from build123d import *

# Parameters (mm, degrees)
SKETCH1_W           = 266
SKETCH1_H           = 7
SKETCH1_R           = 1.8
SKETCH1_W_2         = 15
SKETCH1_H_2         = 166.79
BOSS_EXTRUDE1_DEPTH = 5
SKETCH2_W           = 266
SKETCH2_H           = 9.605
BOSS_EXTRUDE2_DEPTH = 5
SKETCH3_W           = 17.215
SKETCH3_H           = 12.5
SKETCH3_W_2         = 0.785
BOSS_EXTRUDE3_DEPTH = 2
FILLET1_R           = 0.5
FILLET2_R           = 50
FILLET3_R           = 2
FILLET4_R           = 100


with BuildPart() as part:
    # Sketch1 → Boss-Extrude1 (new body)
    # profile 1 of 4: a face of its own
    with BuildSketch(Plane.YZ):
        with Locations((0, 86.895)):
            Rectangle(SKETCH1_W, SKETCH1_H)
        with Locations(Location((113.375, 86.895, 0), (0, 0, 270))):
            Circle(SKETCH1_R, mode=Mode.SUBTRACT)
        with Locations(Location((-113.375, 86.895, 0), (0, 0, 270))):
            Circle(SKETCH1_R, mode=Mode.SUBTRACT)
    # profile 2 of 4: a face of its own
    with BuildSketch(Plane.YZ):
        with Locations((125.5, 0)):
            Rectangle(SKETCH1_W_2, SKETCH1_H_2)
    # profile 3 of 4: a face of its own
    with BuildSketch(Plane.YZ):
        with Locations((-125.5, 0)):
            Rectangle(SKETCH1_W_2, SKETCH1_H_2)
    # profile 4 of 4: a face of its own
    with BuildSketch(Plane.YZ):
        with Locations((0, -86.895)):
            Rectangle(SKETCH1_W, SKETCH1_H)
        with Locations(Location((-113.375, -86.895, 0), (0, 0, 270))):
            Circle(SKETCH1_R, mode=Mode.SUBTRACT)
        with Locations(Location((113.375, -86.895, 0), (0, 0, 270))):
            Circle(SKETCH1_R, mode=Mode.SUBTRACT)
    extrude(amount=BOSS_EXTRUDE1_DEPTH)

    # Sketch2 → Boss-Extrude2 (add)
    with BuildSketch(Plane.YZ.offset(5)):
        with Locations((0, 95.1975)):
            Rectangle(SKETCH2_W, SKETCH2_H)
        with Locations((0, -95.1975)):
            Rectangle(SKETCH2_W, SKETCH2_H)
    extrude(amount=-BOSS_EXTRUDE2_DEPTH)

    # Sketch3 → Boss-Extrude3 (add)
    # profile 1 of 2: a face of its own
    with BuildSketch(Plane(origin=(0, 0, -100), x_dir=(1, 0, 0), z_dir=(0, 0, -1))):
        with Locations((-3.6075, 139.25)):
            Rectangle(SKETCH3_W, SKETCH3_H)
        with BuildLine():
            ThreePointArc((-4.215, 136.45), (-7.015, 139.25), (-4.215, 142.05))
            Line((-4.215, 142.05), (-2.215, 142.05))
            ThreePointArc((-2.215, 142.05), (0.585, 139.25), (-2.215, 136.45))
            Line((-2.215, 136.45), (-4.215, 136.45))
        make_face(mode=Mode.SUBTRACT)
    # profile 2 of 2: a face of its own
    with BuildSketch(Plane(origin=(0, 0, -100), x_dir=(1, 0, 0), z_dir=(0, 0, -1))):
        with Locations((5.3925, 139.25)):
            Rectangle(SKETCH3_W_2, SKETCH3_H)
    extrude(amount=-BOSS_EXTRUDE3_DEPTH)

    # Fillet1
    fillet1_edges = [part.edges().sort_by_distance(p)[0] for p in [
        (2.5, -133, -98),
    ]]
    fillet(fillet1_edges, radius=FILLET1_R)

    # Fillet2
    # the kernel refuses this fillet: 50 mm, written as the material it adds along each edge
    with BuildSketch(Plane(origin=(0, -133, -100), x_dir=(0, 1, 0), z_dir=(0, 0, 1))) as fillet2_piece_1:
        with BuildLine():
            CenterArc((32.745897071, 50), FILLET2_R, 229.086571868, 40.913428132)
            Line((0, 12.215), (0, 0))
            Line((0, 0), (32.745897071, 0))
        make_face()
    extrude(amount=2)

    # Fillet3
    fillet3_edges = [part.edges().sort_by_distance(p)[0] for p in [
        (-12.215, -145.5, -99),
        (5.785, -145.5, -99),
    ]]
    fillet(fillet3_edges, radius=FILLET3_R)

    # Mirror1: part across plane


with BuildPart() as part_1:
    add(part.part)
    add(part.part.mirror(Plane.XY))

    # Mirror2: part across plane


with BuildPart() as part_2:
    add(part_1.part)
    add(part_1.part.mirror(Plane.ZX))

    # Fillet4
    # the kernel refuses this fillet: 100 mm, written as the material it adds along each edge
    with BuildSketch(Plane(origin=(5, 133, 98), x_dir=(1, 0, 0), z_dir=(0, 0, 1)), Plane(origin=(5, 133, -100), x_dir=(1, 0, 0), z_dir=(0, 0, 1)), Plane(origin=(5, -133, -98), x_dir=(1, 0, 0), z_dir=(0, 0, -1)), Plane(origin=(5, -133, 100), x_dir=(1, 0, 0), z_dir=(0, 0, -1))) as fillet4_piece_1:
        with BuildLine():
            CenterArc((100, -12.505349855), FILLET4_R, 172.816154735, 7.183845265)
            Line((0, -12.505349855), (0, 0))
            Line((0, 0), (0.785, 0))
        make_face()
    extrude(amount=2)


solid = part_2.part
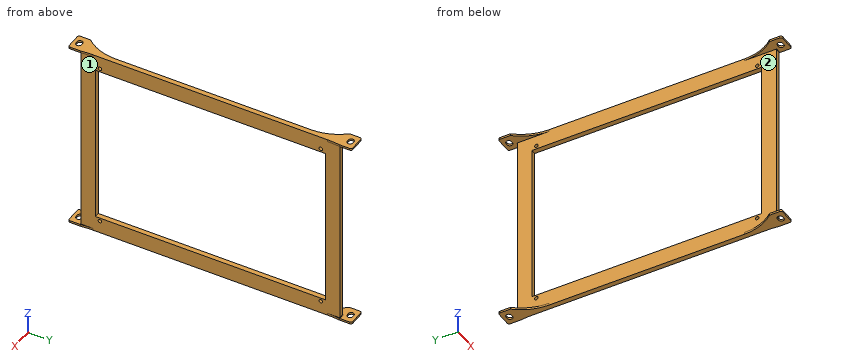
Design review of the part built by this model. Coordinates are the model's own, in mm. Face numbers are marked on the shaded views. Give positions to 0.01 mm unless a question says otherwise; leave off trailing zeros. Order: outer loops, then holes, each group sorted by start corner. A loop starts at its lowest first (then second) coordinate and runs counter-clockwise, first axis right, second up.
1. Add section A-A, the plane z = -5.5. State the section outline as (x, y) points.
Solution:
outline: (0, -133) - (5, -133) - (5, -118) - (0, -118) - close; (0, 118) - (5, 118) - (5, 133) - (0, 133) - close
2. For pin 1 Ø4 at (y, z) = (113.375, 86.895) entering from -X; pin 2 Ø4 at (y, z) = (113.375, -86.895) entering from +X; pin 3 Ø2 at (x, y) = (-1.5, 80) entering from +Z; pin 4 Ø2.5 at (x, z) = (1.5, -34.5) entering from -Y, all flat-tipped, find the tip position at first contact; note any pin that passes through.
Solution:
pin 1: stops at x = 0
pin 2: stops at x = 5
pin 3: passes through
pin 4: stops at y = -133
3. To check wall thickness, follow L1, parallel to Y at x = 1, z = -86.5; L2, parallel to Y at x = 4.25, z = 75.5; L3, parallel to X at y = -129, z = -9.5. State the ranges of each line that lie inside material, in increasing order.
Solution:
L1: y = -133 to -115.13, -111.62 to 111.62, 115.13 to 133
L2: y = -133 to -118, 118 to 133
L3: x = 0 to 5
4. Add section B-B, the plane y = -6. State the section outline as (x, z) points (3 decimals), then the cut area to 3 significant figures.
Solution:
outline: (0, -100) - (5, -100) - (5, -83.395) - (0, -83.395) - close; (0, 83.395) - (5, 83.395) - (5, 100) - (0, 100) - close
area: 166 mm2
5. Mouldability with a two-part tool opening along Z and no side actions: class the marked faces 1 and 2 as +Z half, -Z half, draft (parallel to the pull), parting line (faces both ways), or undercut.
Solution:
face 1: undercut
face 2: undercut
